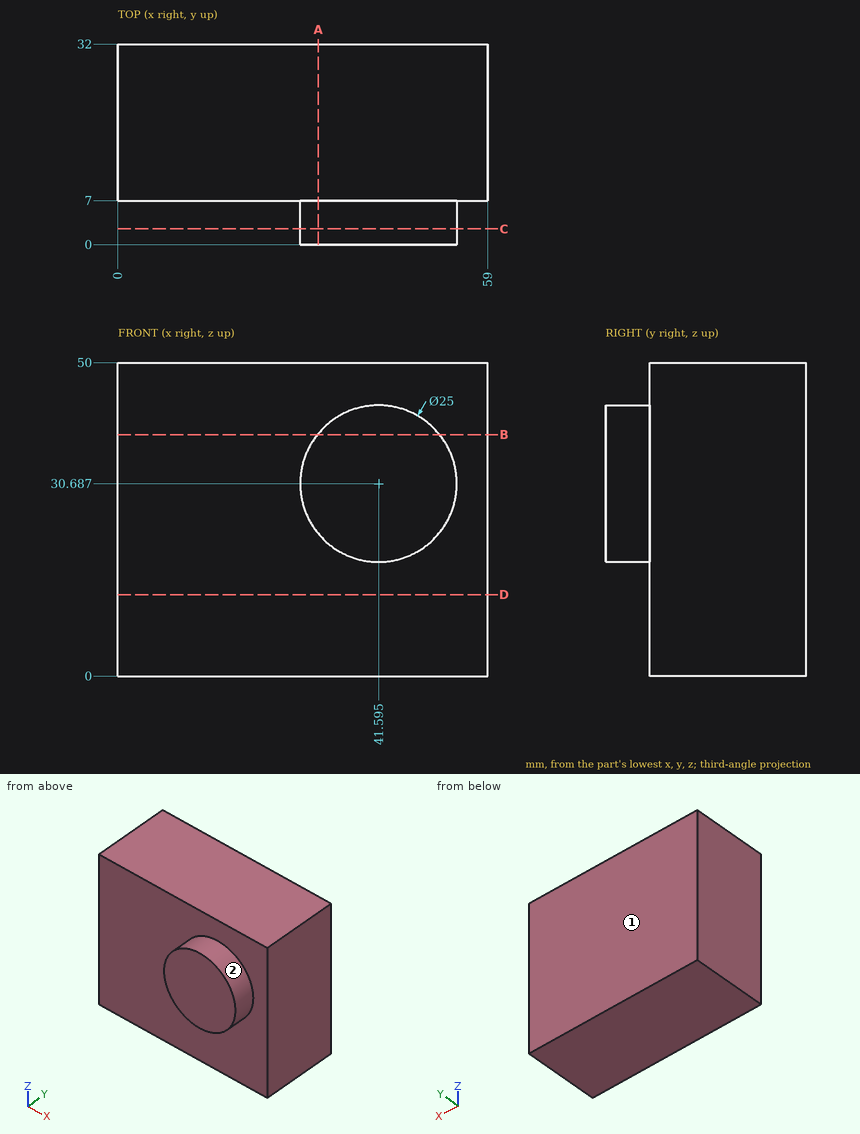
Could you check a few things on this drawing? It's one solid part, dimensions in mm from its lowest x, y, z. A direction names the side the tool comes from. Give positions to 0.01 mm unless a question says otherwise; leave off trailing zeros. Write each loop counter-clockwise with the first axis right and the second up, starting at its lowest first coordinate (ties: lowest second). Pieces come first, ordered by that corner, then holes.
(1) On a 3-axis mill with a long thin cutter (end or side, diameter ignored), from which of +Z, -Z, +X, -X, +Y, -Y can I reach the whole of each face in a straight line? I mean the marked faces 1 and 2. Say none if no direction works.
Output values:
face 1: +Z, -Z, +X, -X, +Y
face 2: -Y
(2) Imagine slicing it at D-D, the plane z = 13. Write out the boundary of the cut face in (x, y).
Output values:
outline: (0, 7) - (59, 7) - (59, 32) - (0, 32) - close
(3) Imagine slicing it at B-B, the plane z = 38.5. Write out the boundary of the cut face in (x, y).
Output values:
outline: (0, 7) - (31.84, 7) - (31.84, 0) - (51.35, 0) - (51.35, 7) - (59, 7) - (59, 32) - (0, 32) - close
(4) Imagine slicing it at A-A, the plane x = 32. Write out the boundary of the cut face in (y, z) (1 decimal), and give its area (3 significant figures).
Output values:
outline: (0, 22.7) - (7, 22.7) - (7, 0) - (32, 0) - (32, 50) - (7, 50) - (7, 38.7) - (0, 38.7) - close
area: 1,360 mm2
(5) Imagine slicing it at C-C, the plane y = 2.5. Write out the boundary of the cut face in (x, z) (1 decimal), and give its area (3 significant figures).
Output values:
outline: circle Ø25 at (41.6, 30.7)
area: 491 mm2
(6) If I drill on L1, parallel to Y at x = 19, z = 33.5; L2, parallel to X at y = 6, z = 34, over which ranges is the centre line in solid material (lowest first)?
Output values:
L1: y = 7 to 32
L2: x = 29.54 to 53.65
